Autodesk Inventor part; units mm, degrees
ref_plane "C_XY" through (10.1565, 1.75, 0) normal (0, 0, 1) x (1, 0, 0)
ref_plane "C_YZ" through (10.1565, 1.75, 0) normal (1, 0, 0) x (0, 1, 0)
ref_plane "C_ZX" through (10.1565, 1.75, 0) normal (0, 1, 0) x (0, 0, 1)
sketch "Sketch_1" plane through (0, 0, 0) normal (0, 0, 1) x (1, 0, 0)
  line L0 (0, 1) -> (0, 0)
  line L1 (0, 0) -> (10.25, 0)
  arc A0 (10.25, 0) -> (11.4874, 2.9874) centre (10.25, 1.75) ccw
  line L2 (11.4874, 2.9874) -> (9.2749, 5.2)
  line L3 (9.2749, 5.2) -> (8.5678, 4.4929)
  line L4 (8.5678, 4.4929) -> (10.7803, 2.2803)
  arc A1 (10.25, 1) -> (10.7803, 2.2803) centre (10.25, 1.75) ccw
  line L5 (10.25, 1) -> (0, 1)
extrude "Extrusion1" add sketch "Sketch_1" along normal mid plane 18
sketch "Sketch_2" plane through (0, 0, 0) normal (0, 1, 0) x (-1, 0, 0)
  line L0 (2, 11) -> (-16, 11)
  line L1 (-16, 11) -> (-16, -12)
  line L2 (-16, -12) -> (2, -12)
  line L3 (2, -12) -> (2, 11)
  line L4 (0, -7) -> (0, 7)
  arc A0 (0, 7) -> (-4, 7) centre (-2, 7) ccw
  line L5 (-4, 7) -> (-4, 4.75)
  line L6 (-4, 4.75) -> (-12, 4.75)
  line L7 (-12, 4.75) -> (-12, -4.75)
  line L8 (-12, -4.75) -> (-4, -4.75)
  line L9 (-4, -4.75) -> (-4, -7)
  arc A1 (-4, -7) -> (0, -7) centre (-2, -7) ccw
extrude "Extrusion2" cut sketch "Sketch_2" along normal mid plane 18
sketch "Sketch_3" plane through (0, 0, 0) normal (0, 1, 0) x (-1, 0, 0)
  circle A0 centre (-2, -7) radius 1.05
extrude "Extrusion3" cut sketch "Sketch_3" along normal mid plane 18
sketch "Sketch_4" plane through (0, 0, 0) normal (0, 1, 0) x (-1, 0, 0)
  circle A0 centre (-2, 7) radius 1.05
extrude "Extrusion4" cut sketch "Sketch_4" along normal mid plane 18
ref_plane "C_XY" through (10.1565, 1.75, 0) normal (0, 0, 1) x (1, 0, 0)
ref_plane "C_YZ" through (10.1565, 1.75, 0) normal (1, 0, 0) x (0, 1, 0)
ref_plane "C_ZX" through (10.1565, 1.75, 0) normal (0, 1, 0) x (0, 0, 1)
properties part number "PKWS1_s"
For this review, take the finished solid that the model builds, in its own axes (mm). A direction names the side the tool comes from. Round coordinates to 2 decimals unless told otherwise and drop trailing zeros. Write each loop counter-clockwise with the first axis right and the second up, starting at its lowest first coordinate (ties: lowest second). Pieces come first, ordered by that corner, then holes. Notation, with made-up numbers: M 71,65 L 112,65 A8 ccw 112,78 Z; hole C 83.25,42.5 d5. An arc over 180 degrees is marked long. Write item = value, one per line. Start each with the question number.
(1) For line 1 along Z through (x, y) = (2, 0.4); line 2 along X through (y, z) = (0.7, 7); line 3 along Y through (x, z) = (1, -3), list the stretches that pass through material, from the lowest coordinate up.
(2) For faces 1 (the face through (4, 1, 0)), 2 (the face through (4, 0.5, 5.9)), 3 (the face through (9.2, 0.85, -4.75)), 4 (the face through (0, 0.5, -0.1)), 5 (the face through (2.14, 0.49, 5.96)), list the 3-axis set-ups (+Z, -Z, +X, -X, +Y, -Y) from which the entire face can be reached by the end or side of a thin tool; tool diameter is ignored.
(3) We need section C-C (y = 0.55). Give the boundary of the cut face in (x, z).
(4) The part is to be moulded in two halves that separate along Y. For faces 6 (the face through (8.57, 0.85, 4.75)), 7 (the face through (10.397, 4.078, -0.067)), 8 (the face through (9.66, 3.4, -0.07)), say which applies: +Y half, -Y half, draft (parallel to the pull), parting line (faces both ways), or undercut.
(5) We need section B-B (z = 3). Give the boundary of the cut face in (x, y), then the cut area to 3 significant figures.
(6) We need section A-A (x = 2). Give the boundary of the cut face in (y, z).
(7) We need section D-D (x = 9.5). Give the boundary of the cut face in (y, z).
(8) Clearance check with flat-ended pins moving along their axes: pin 1 Ø0.5 at (y, z) = (0.5, 6.5) entering from +X; pin 2 Ø1.9 at (x, z) = (2, 7) entering from -Y; pin 3 Ø3.5 at (x, z) = (2, -7) entering from +Y. State where each tip first meets the part, or that it passes through.
Results found:
q1.line_1 = -9 to -8.05, -5.95 to 5.95, 8.05 to 9
q1.line_2 = 0 to 0.95, 3.05 to 4
q1.line_3 = 0 to 1
q2.face_1 = +Z, -Z, -X
q2.face_2 = +Z, +X, +Y, -Y
q2.face_3 = -Z, +X, +Y, -Y
q2.face_4 = +Z, -Z, -X, +Y, -Y
q2.face_5 = +Y, -Y
q3.outline = M 0,-7 A2 ccw 4,-7 L 4,-4.75 L 11.52,-4.75 L 11.52,4.75 L 4,4.75 L 4,7 A2 ccw 0,7 Z; hole C 2,-7 d2.1; hole C 2,7 d2.1
q4.face_6 = draft
q4.face_7 = +Y half
q4.face_8 = undercut
q5.outline = M 0,0 L 10.25,0 A1.75 ccw 11.49,2.99 L 9.27,5.2 L 8.57,4.49 L 10.78,2.28 A0.75 cw 10.25,1 L 0,1 Z
q5.area = 16.3 mm²
q6.outline = M 0,-9 L 1,-9 L 1,-8.05 L 0,-8.05 Z; M 0,-5.95 L 1,-5.95 L 1,5.95 L 0,5.95 Z; M 0,8.05 L 1,8.05 L 1,9 L 0,9 Z
q7.outline = M 0,-4.75 L 1,-4.75 L 1,4.75 L 0,4.75 Z; M 3.56,-4.75 L 4.97,-4.75 L 4.97,4.75 L 3.56,4.75 Z
q8.pin_1 = 4
q8.pin_2 = through
q8.pin_3 = 1
